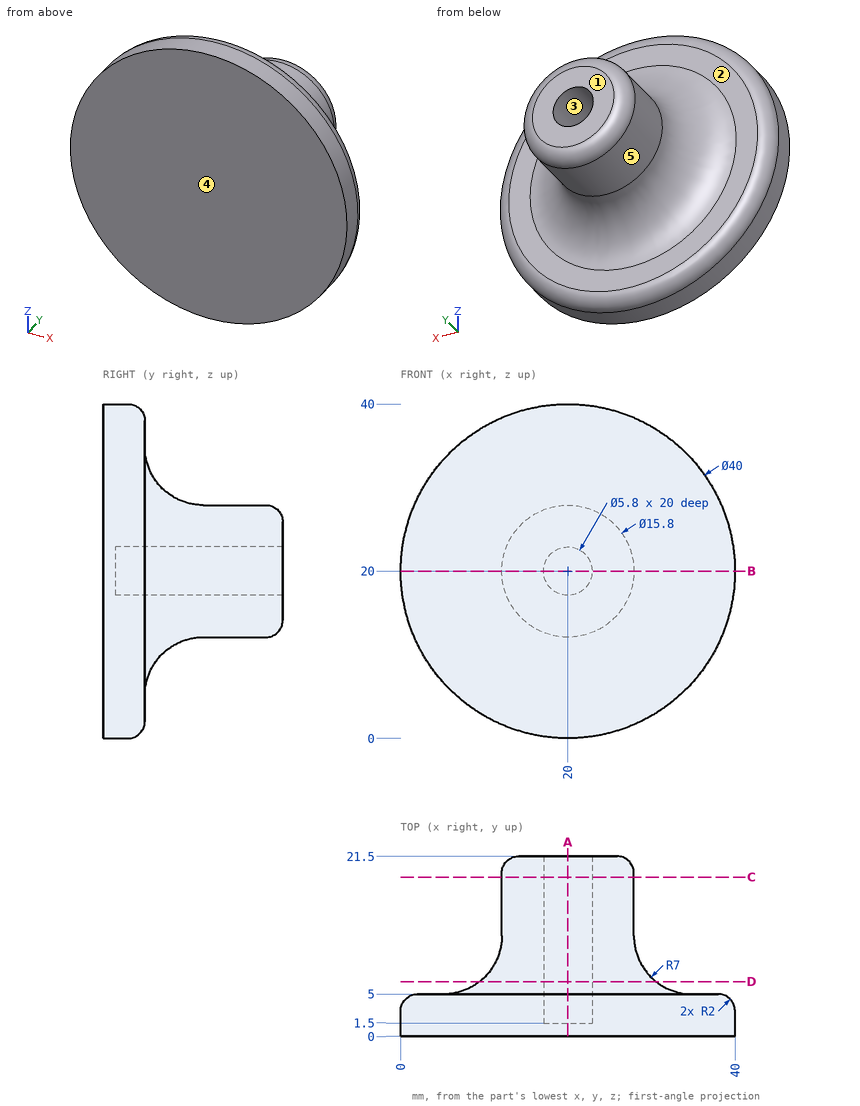
The drawing under review shows one solid part. Ordinate dimensions are in mm from its lowest x, y, z. A direction names the side the tool comes from. Give positions to 0.01 mm unless a question says otherwise; leave off trailing zeros. Write each loop counter-clockwise with the first axis right and the second up, starting at its lowest first coordinate (ties: lowest second). Pieces come first, ordered by that corner, then holes. Notation, with made-up numbers: M 85.5,34 L 106.5,34 A32 cw 106.5,71 Z; hole C 44.25,-26.5 d4. An arc over 180 degrees is marked long. Write each question's results on one line, items separated by ' | '. Start each with the question number.
1. We need section C-C (y = 19). Write out the cut boundary in (x, z), and give its area (3 significant figures).
2. We need section D-D (y = 6.5). Write out the cut boundary in (x, z), and give its area (3 significant figures).
3. We need section B-B (z = 20). Write out the cut boundary in (x, y).
4. For probe 1 along X at (y, z) = (16, 20); probe 2 along Y at (x, z) = (16, 2.5), list the stretches that pass through material, from the lowest coordinate up. Write a range as [from, to].
5. We need section A-A (x = 20). Write out the cut boundary in (y, z).
6. Insertion check: pin 1 Ø12 at (x, y) = (34, 14.5) entering from +Z; pin 2 Ø12 at (y, z) = (14.5, 16.5) entering from +X; pin 3 Ø5 at (x, z) = (19.5, 9) entering from +Y; pin 4 Ø3 at (x, z) = (19, 20) entering from +Y. Each pin has a flat end and moves straight along its axis. Give the tip position at first contact, or say it passes through.
7. Mouldability with a two-part tool opening along Z and no side actions: class the marked faces 3, 4 and 5 as released by +Z, released by -Z, zero draft, split by the parting line, or undercut.
8. For the marked faces 1 and 2, list the 3-axis set-ups (+Z, -Z, +X, -X, +Y, -Y) from which the entire face can be reached by the end or side of a thin tool; tool diameter is ignored.
Results found:
1) outline: C 20,20 d15.8; hole C 20,20 d5.8 | area: 170 mm^2
2) outline: C 20,20 d21.14; hole C 20,20 d5.8 | area: 325 mm^2
3) outline: M 0,0 L 40,0 L 40,3 A2 ccw 38,5 L 34.9,5 A7 cw 27.9,12 L 27.9,19.5 A2 ccw 25.9,21.5 L 22.9,21.5 L 22.9,1.5 L 17.1,1.5 L 17.1,21.5 L 14.1,21.5 A2 ccw 12.1,19.5 L 12.1,12 A7 cw 5.1,5 L 2,5 A2 ccw 0,3 Z
4) probe 1: x = [12.1, 17.1], [22.9, 27.9] | probe 2: y = [0, 5]
5) outline: M 0,0 L 3,0 A2 ccw 5,2 L 5,5.1 A7 cw 12,12.1 L 19.5,12.1 A2 ccw 21.5,14.1 L 21.5,17.1 L 1.5,17.1 L 1.5,22.9 L 21.5,22.9 L 21.5,25.9 A2 ccw 19.5,27.9 L 12,27.9 A7 cw 5,34.9 L 5,38 A2 ccw 3,40 L 0,40 Z
6) pin 1: passes through | pin 2: stops at x = 28.52 | pin 3: stops at y = 9.14 | pin 4: stops at y = 1.5
7) face 3: undercut | face 4: zero draft | face 5: split by the parting line
8) face 1: +Z, -Z, +X, -X, +Y | face 2: +Y
